```python
from build123d import *

# Parameters (mm, degrees)
FURO_COM_FOLGA_DE_M61_D = 6.6


with BuildPart() as part:
    # Esboço1 → Revolução1 (revolve)
    with BuildSketch(Plane(origin=(0, 0, 0), x_dir=(0, 0, -1), z_dir=(1, 0, 0))):
        with BuildLine():
            Line((0, 0), (0, 6.5))
            Line((0, 6.5), (1.5, 6.5))
            Line((1.5, 6.5), (1.5, 4.5))
            Line((1.5, 4.5), (3.1, 4.5))
            ThreePointArc((3.1, 4.5), (4.1, 5.5), (5.1, 4.5))
            Line((5.1, 4.5), (10.6, 4.5))
            ThreePointArc((10.6, 4.5), (10.953553391, 4.353553391), (11.1, 4))
            Line((11.1, 4), (11.1, 0))
            Line((11.1, 0), (0, 0))
        make_face()
    revolve(axis=Axis((0, 0, -11.1), (0, 0, 1)))

    # Furo com folga de M61 (through all)
    with Locations(Plane.XY):
        with Locations((0, 0)):
            Hole(FURO_COM_FOLGA_DE_M61_D / 2)


solid = part.part
```
Design review of the part built by this model. Coordinates are the model's own, in mm. A direction names the side the tool comes from. Give positions to 0.01 mm unless a question says otherwise; leave off trailing zeros. Order: outer loops, then holes, each group sorted by start corner. A loop starts at its lowest first (then second) coordinate and runs counter-clockwise, first axis right, second up. Notation, with made-up numbers: (50, -16.75) -> (68, -16.75) arc R20 ccw to (68, 22.25) -> close; hole circle Ø9 at (68.5, 86). An arc over 180 degrees is marked (long way). Write each question's results on one line, items separated by ' | '. Start each with the question number.
Q1. Wall thickness on L1, parallel to Y at x = 0, z = -4; L2, parallel to Y at x = 0, z = -5.25; L3, parallel to Z at x = -4.5, y = -3.5: over which ranges is each line inside the solid? List them lowest first. Write a range as from..to.
Q2. Add section C-C on z = -8.5. Give the boundary of the cut face in (x, y), and give its area (3 significant figures).
Q3. Add section A-A on x = 0. Give the boundary of the cut face in (y, z), and give its area (3 significant figures).
Q4. For pin 1 (3 mm diameter, centred on x = -4.5, z = -3.5, fed in from +Y); pin 2 (6 mm diameter, centred on x = 2.5, z = -8.5, fed in from -Y); pin 3 (4 mm diameter, centred on x = -3, z = -9, fed in from -Y), all flat-tipped, find the tip position at first contact; note any pin that passes through.
Q5. Machinability: for faces 1 (the cylindrical face through (2.43, 2.23, -5.63)), 2 (the cylindrical face through (-4.46, -0.59, -2.31)), which of the approach directions +Z, -Z, +X, -X, +Y, -Y give a long, thin tool a straight path to every point of the face, cutting with its end or side? Answer none if there is none.
Q6. Mouldability with a two-part tool opening along Z and no side actions: class faces 3 (the flat face through (-3, -2, -11.1)), 4 (the cylindrical face through (-4.46, -0.59, -7.89)), 5 (the flat face through (-2, 3, 0)), 6 (the flat face through (-4.42, -1.54, -1.5)) as +Z half, -Z half, draft (parallel to the pull), parting line (faces both ways), or undercut.
Found:
1) L1: y = -5.49..-3.3, 3.3..5.49 | L2: y = -4.5..-3.3, 3.3..4.5 | L3: z = -1.5..0
2) outline: circle Ø9 at (0, 0); hole circle Ø6.6 at (0, 0) | area: 29.4 mm2
3) outline: (-6.5, -1.5) -> (-4.5, -1.5) -> (-4.5, -3.1) arc R1 ccw to (-4.5, -5.1) -> (-4.5, -10.6) arc R0.5 ccw to (-4, -11.1) -> (-3.3, -11.1) -> (-3.3, 0) -> (-6.5, 0) -> close; (3.3, -11.1) -> (4, -11.1) arc R0.5 ccw to (4.5, -10.6) -> (4.5, -5.1) arc R1 ccw to (4.5, -3.1) -> (4.5, -1.5) -> (6.5, -1.5) -> (6.5, 0) -> (3.3, 0) -> close | area: 35.7 mm2
4) pin 1: stops at y = 4.55 | pin 2: stops at y = -4.5 | pin 3: stops at y = -4.39
5) face 1: +Z, -Z | face 2: none
6) face 3: -Z half | face 4: draft | face 5: +Z half | face 6: undercut
